Check sheet for the modelled part. Datum: model origin and axes. Units: mm. A direction names the side the tool comes from. Coordinates: 2 decimals unless noted, no trailing zeros. Write each loop counter-clockwise with the first axis right and the second up, starting at its lowest first coordinate (ties: lowest second). Pieces come first, ordered by that corner, then holes. Notation, with made-up numbers: (24.25, 41) - (49.25, 41) arc R30 cw to (49.25, 63) - close; hole circle Ø9 at (28.25, 19.5). An arc over 180 degrees is marked (long way). Write each question's results on one line, items separated by ' | '.
Autodesk Inventor part; units mm, degrees
ref_plane "XZ Plane" through (0, 0, 0) normal (0, 1, 0) x (-1, 0, 0)
ref_plane "XY Plane" through (0, 0, 0) normal (0, 0, 1) x (1, 0, 0)
sketch "Sketch1" plane through (0, 0, 0) normal (0, 1, 0) x (-1, 0, 0)
  line L0 (-209.55, 254) -> (-209.55, -254)
  line L1 (-209.55, -254) -> (209.55, -254)
  line L2 (209.55, -254) -> (209.55, 254)
  line L3 (209.55, 254) -> (-209.55, 254)
  line L4 (-209.55, 254) -> (209.55, -254) construction
  line L5 (-209.55, -254) -> (209.55, 254) construction
  point P0 (0, 0)
  dimension "baseLength" = 508
  dimension "baseWidth" = 419.1
extrude "Extrusion1" add sketch "Sketch1" along normal blind 19.05
sketch "Sketch2" plane through (0, 0, 0) normal (0, -1, 0) x (1, 0, 0)
  line L0 (209.55, 254) -> (209.55, -254)
  line L1 (209.55, 177.8) -> (158.75, 177.8)
  line L2 (158.75, 177.8) -> (158.75, 25.4)
  line L3 (158.75, 25.4) -> (209.55, 25.4)
  line L4 (209.55, 25.4) -> (209.55, 177.8)
  line L5 (-209.55, 254) -> (209.55, 254)
  point P0 (0, 0)
  dimension "backToEndOfGearBox" = 76.2
  dimension "backToFrontOfGearBox" = 228.6
  dimension "wdithForGearBox" = 50.8
extrude "Extrusion2" cut sketch "Sketch2" against normal through all
mirror "Mirror1" about plane through (0, 0, 0) normal (1, 0, 0) of "Extrusion2"
properties part number "BasePlate" material "Wood (Walnut)"
1. Sectioned sample at A-A (x = -168.5). Record the cut outline in (y, z), then the cut area to 3 significant figures.
Values follow:
outline: (0, -254) - (19.05, -254) - (19.05, 25.4) - (0, 25.4) - close; (0, 177.8) - (19.05, 177.8) - (19.05, 254) - (0, 254) - close | area: 6,770 mm^2
2. Access from +Z, -Z, +X, -X, +Y, -Y to the whole of each face (thin tool, end or side, straight path). Record for faces 1 (the flat face through (-184, 9, 177.8)), 2 (the flat face through (184, 9, 25.4)), 3 (the flat face through (-209.55, 9, -116)).
Values follow:
face 1: -X, +Y, -Y | face 2: +X, +Y, -Y | face 3: +Z, -Z, -X, +Y, -Y
3. Sectioned sample at B-B (y = 9.75). Record the cut outline in (x, z), then the cut area to 3 significant figures.
Values follow:
outline: (-209.55, -254) - (209.55, -254) - (209.55, 25.4) - (158.75, 25.4) - (158.75, 177.8) - (209.55, 177.8) - (209.55, 254) - (-209.55, 254) - (-209.55, 177.8) - (-158.75, 177.8) - (-158.75, 25.4) - (-209.55, 25.4) - close | area: 197,000 mm^2
4. Go/stop test with flat-tipped pins: pin 1 (9.5 mm diameter, centred on y = 9, z = 133, fed in from -X); pin 2 (12 mm diameter, centred on x = 161.5, z = -185.5, fed in from -Y); pin 3 (5.5 mm diameter, centred on y = 5.5, z = 100, fed in from +X). Record where each tip stops, or that it passes through.
Values follow:
pin 1: stops at x = -158.75 | pin 2: stops at y = 0 | pin 3: stops at x = 158.75
5. Sectioned sample at C-C (z = 118). Record the cut outline in (x, y), then the cut area to 3 significant figures.
Values follow:
outline: (-158.75, 0) - (158.75, 0) - (158.75, 19.05) - (-158.75, 19.05) - close | area: 6,050 mm^2
6. Material ranges on L1, parallel to X at y = 5, z = 70.5, recorded low to high. Write a range as [from, to].
Values follow:
L1: x = [-158.75, 158.75]
7. Draft check along Z on faces 4 (the flat face through (-185, 9, 25.4)), 5 (the flat face through (-3, 9, 254)), 6 (the flat face through (158.75, 9, 103)), 7 (the flat face through (3, 0, 4)). Enter one of: pulls with the +Z half, pulls with the -Z half, needs draft (parallel to the pull), parting line crosses it, or undercut.
Values follow:
face 4: undercut | face 5: pulls with the +Z half | face 6: undercut | face 7: needs draft
